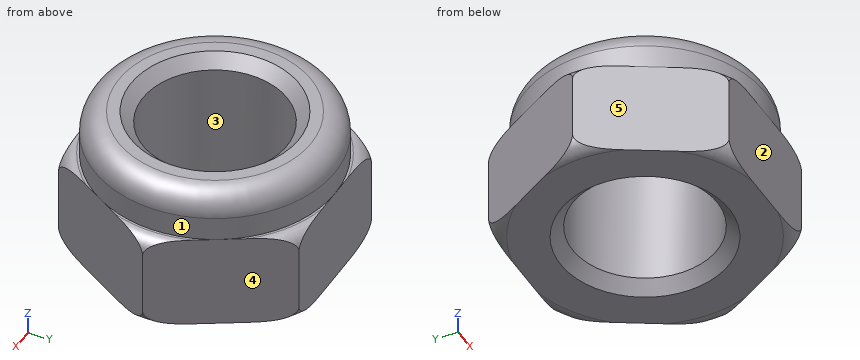
```python
from build123d import *

# Parameters (mm, degrees)
SZKIC1_R                    = 3
DODANIE_WYCI_GNI_CIE1_DEPTH = 4
SZKIC2_R                    = 5
SZKIC2_R_2                  = 3
DODANIE_WYCI_GNI_CIE2_DEPTH = 6
SFAZOWANIE1_SIZE            = 0.5


with BuildPart() as part:
    # Szkic1 → Dodanie-wyciągnięcie1 (new body)
    with BuildSketch(Plane.XY):
        Polygon((-5.773502692, 0), (-2.886751346, -5), (2.886751346, -5), (5.773502692, 0), (2.886751346, 5), (-2.886751346, 5), align=None)
        Circle(SZKIC1_R, mode=Mode.SUBTRACT)
    extrude(amount=DODANIE_WYCI_GNI_CIE1_DEPTH)

    # Szkic2 → Dodanie-wyciągnięcie2 (add)
    with BuildSketch(Plane.XY):
        Circle(SZKIC2_R)
        Circle(SZKIC2_R_2, mode=Mode.SUBTRACT)
    extrude(amount=DODANIE_WYCI_GNI_CIE2_DEPTH)

    # Sfazowanie1
    sfazowanie1_edges = [part.edges().sort_by_distance(p)[0] for p in [
        (-3, 0, 0),
        (-3, 0, 6),
    ]]
    chamfer(sfazowanie1_edges, length=SFAZOWANIE1_SIZE)

    # Szkic3 → Wycięcie-obrót1 (revolve, cut)
    with BuildSketch(Plane(origin=(0, 0, 0), x_dir=(1, 0, 0), z_dir=(0, 1, 0))):
        with BuildLine():
            Line((-5.773502692, 0), (-5.773502692, -0.673502692))
            ThreePointArc((-5.773502692, -0.673502692), (-5.576238321, -0.197264371), (-5.1, 0))
            Line((-5.1, 0), (-5.773502692, 0))
        make_face()
        with BuildLine():
            ThreePointArc((-5.1, -4), (-5.576238321, -3.802735629), (-5.773502692, -3.326497308))
            Line((-5.773502692, -3.326497308), (-5.773502692, -4))
            Line((-5.773502692, -4), (-5.1, -4))
        make_face()
        with BuildLine():
            Line((-5, -6), (-4, -6))
            ThreePointArc((-4, -6), (-4.707106781, -5.707106781), (-5, -5))
            Line((-5, -5), (-5, -6))
        make_face()
    revolve(axis=Axis((0, 0, -1.701574894), (0, 0, 1)), mode=Mode.SUBTRACT)


solid = part.part
```
Here's how the part is built. I have some questions about the finished solid (model axes, mm). Face numbers are marked on the shaded views. A direction names the side the tool comes from. Give positions to 0.01 mm unless a question says otherwise; leave off trailing zeros. Use one line per item in the form item = value. Start each with the question number.
1) Thinking about a two-plate mould opening in Y: for the marked faces 3, 4 and 5, which applies, +Y half, -Y half, draft (parallel to the pull), parting line (faces both ways), or undercut?
2) For P1, Ø1.5, axis at x = -0.5, y = -1, coming from the +Z side; P2, Ø0.7, axis at x = 3, y = -4.5, coming from the +Z side; P3, Ø0.8, axis at x = 5, y = 0.5, coming from the +Z side, each with a flat end and sliding along its axis, tell me the tip position at first contact or that it passes through.
3) Please list where these lines run through material, in increasing order: line 1 along Y through (x, z) = (0, 3.35); line 2 along Z through (x, y) = (-4, -0.75); line 3 along X through (y, z) = (2.5, 2.75).
4) Which directions (+Z, -Z, +X, -X, +Y, -Y) give clear straight access to the entire face, cutting with the end or side of a thin tool? Please do the marked faces 1 and 2.
Check values:
q1.face_3 = undercut
q1.face_4 = +Y half
q1.face_5 = -Y half
q2.P1 = through
q2.P2 = 4
q2.P3 = 5.78
q3.line_1 = -5 to -3, 3 to 5
q3.line_2 = 0 to 6
q3.line_3 = -4.33 to -1.66, 1.66 to 4.33
q4.face_1 = +Z
q4.face_2 = +Z, -Z, +X, -X, -Y
